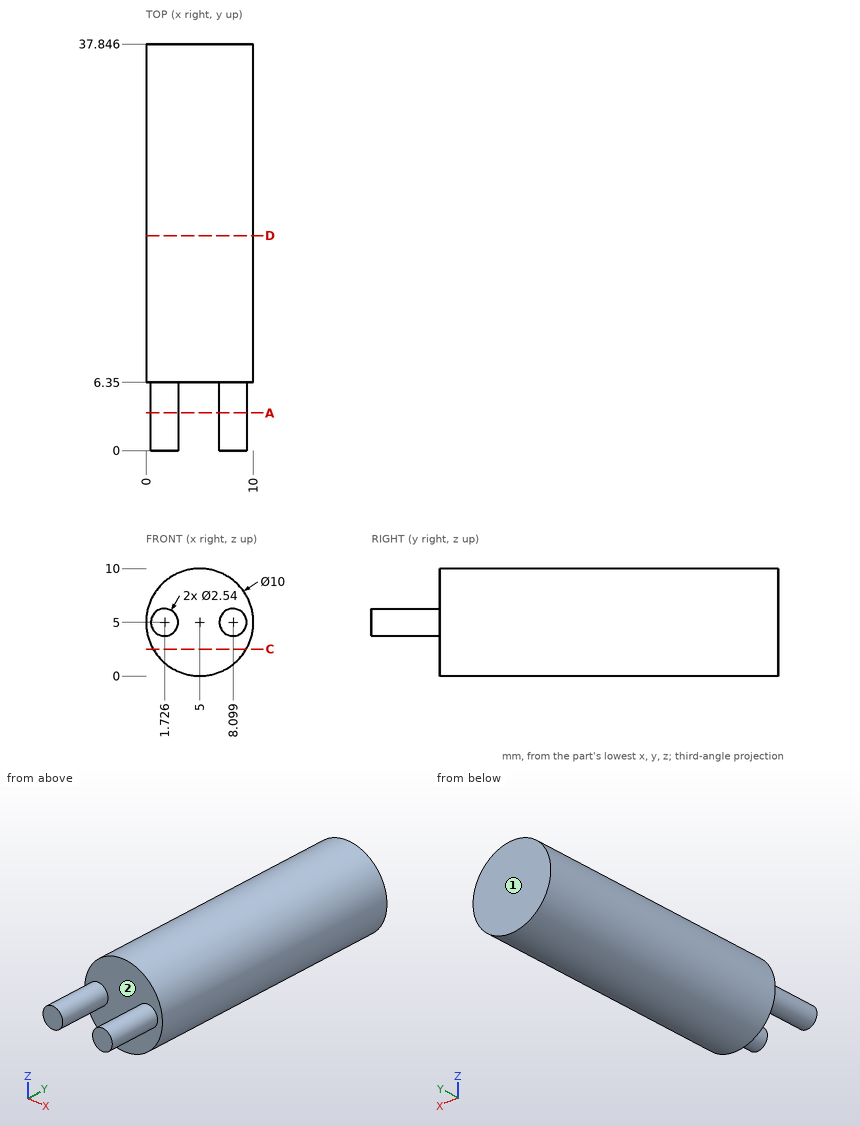
Could you check a few things on this drawing? It's one solid part, dimensions in mm from its lowest x, y, z. A direction names the side the tool comes from. Give positions to 0.01 mm unless a question says otherwise; leave off trailing zeros. Order: outer loops, then holes, each group sorted by start corner. A loop starts at its lowest first (then second) coordinate and runs counter-clockwise, first axis right, second up. Notation, with made-up numbers: (51, 87) - (64, 87) arc R27 ccw to (64, 118) - close; hole circle Ø5 at (19.25, 18.25). An arc over 180 degrees is marked (long way). Answer as a JSON object with one key per item and string values. Group by question number.
Item 1: Which directions (+Z, -Z, +X, -X, +Y, -Y) give clear straight access to the entire face, cutting with the end or side of a thin tool? Please do the marked faces 1 and 2.
Item 2: For P1, Ø1.5, axis at x = 6.5, y = 12.5, coming from the +Z side; P2, Ø1, axis at x = 9, y = 4.5, coming from the -Z side (1 decimal), each with a flat end and sliding along its axis, tell me the tip position at first contact or that it passes through.
Item 3: If we section it at A-A on y = 3.5: Please give me the cut outline in (x, z).
Item 4: If we section it at D-D on y = 20: Please give me the cut outline in (x, z).
Item 5: Please list where these lines run through material, in increasing order: probe 1 along Y at (x, z) = (3.25, 3.25); probe 2 along X at (y, z) = (22.5, 4.75); probe 3 along X at (y, z) = (3, 4) (1 decimal).
Item 6: If we section it at C-C on z = 2.5: Please give me the cut outline in (x, y), and give its area (3 significant figures).
Result set:
{
 "1": {"face 1": "+Z, -Z, +X, -X, +Y", "face 2": "-Y"},
 "2": {"P1": "z = 9.94", "P2": "z = 3.8"},
 "3": {"outline": "circle Ø2.54 at (1.73, 5); circle Ø2.54 at (8.1, 5)"},
 "4": {"outline": "circle Ø10 at (5, 5)"},
 "5": {"probe 1": "6.35 to 37.85", "probe 2": "0.01 to 9.99", "probe 3": "0.9 to 2.5, 7.3 to 8.9"},
 "6": {"outline": "(0.67, 6.35) - (9.33, 6.35) - (9.33, 37.85) - (0.67, 37.85) - close", "area": "273 mm²"}
}
